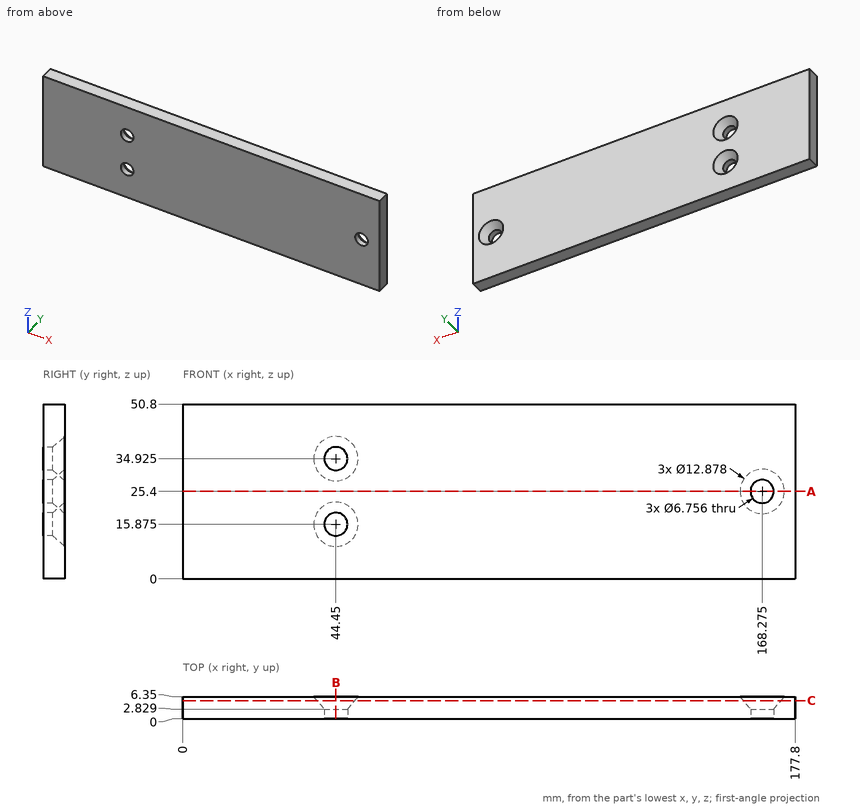
Could you check a few things on this drawing? It's one solid part, dimensions in mm from its lowest x, y, z. Give positions to 0.01 mm unless a question says otherwise; leave off trailing zeros. Order: outer loops, then holes, each group sorted by start corner. A loop starts at its lowest first (then second) coordinate and runs counter-clockwise, first axis right, second up. Notation, with made-up numbers: (-32.5, 36.5) - (10.5, 36.5) arc R19 ccw to (10.5, 43.5) - close; hole circle Ø10 at (-32.75, 72). An arc over 180 degrees is marked (long way). Return JSON: item names as keys, results as strings. Group by question number.
Q1. Suppose I cut it at A-A, the plane z = 25.4. Please give me the cut outline in (x, y), and give its area (3 significant figures).
Q2. Will these pins go through, and if not, where does the flat tip stop? pin 1 Ø8 at (x, z) = (168.275, 25.4) entering from +Y (1 decimal); pin 2 Ø6 at (x, z) = (44.45, 34.925) entering from -Y.
Q3. Suppose I cut it at B-B, the plane x = 44.45. Please give me the cut outline in (y, z), and give its area (3 significant figures).
Q4. Please list where these lines run through material, in increasing order: line 1 along Z through (x, y) = (44.45, 0.8); line 2 along Z through (x, y) = (40.5, 5.75); line 3 along X through (y, z) = (6.25, 36). Write a range as [from, to].
Q5. Suppose I cut it at C-C, the plane y = 5.25. State how many separate pieces and enclosed holes the cut face has, and give its area (3 significant figures).
Resolved:
{
 "1": {"outline": "(0, 0) - (164.9, 0) - (164.9, 2.83) - (161.84, 6.35) - (0, 6.35) - close; (171.65, 0) - (177.8, 0) - (177.8, 6.35) - (174.71, 6.35) - (171.65, 2.83) - close", "area": "1,080 mm2"},
 "2": {"pin 1": "stops at y = 3.5", "pin 2": "passes through"},
 "3": {"outline": "(0, 0) - (6.35, 0) - (6.35, 9.44) - (2.83, 12.5) - (0, 12.5) - close; (0, 19.25) - (2.83, 19.25) - (6.35, 22.31) - (6.35, 28.49) - (2.83, 31.55) - (0, 31.55) - close; (0, 38.3) - (2.83, 38.3) - (6.35, 41.36) - (6.35, 50.8) - (0, 50.8) - close", "area": "215 mm2"},
 "4": {"line 1": "z = [0, 12.5], [19.25, 31.55], [38.3, 50.8]", "line 2": "z = [0, 11.47], [20.28, 30.52], [39.33, 50.8]", "line 3": "x = [0, 38.19], [50.71, 177.8]"},
 "5": {"separate pieces": "1", "enclosed holes": "3", "area": "8,750 mm2"}
}
